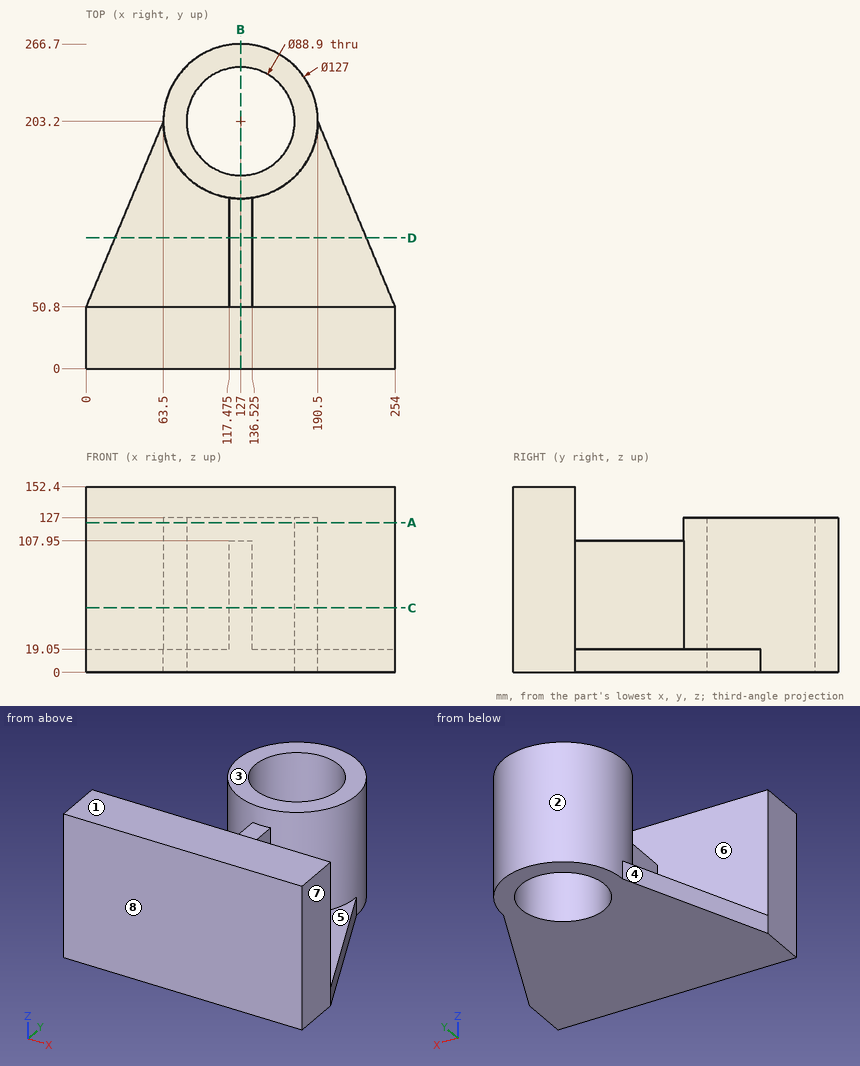
Source: three-view drawing plus pictorial views. Frame: mm from the lowest corner of the part. A direction names the side the tool comes from. Round coordinates to 2 decimals unless told otherwise and drop trailing zeros. Loops run counter-clockwise (first coordinate to the right, second up) from the corner with the lowest first, then second, coordinate; pieces in that order, holes last.
Q1. Section D-D, the plane y = 107.5. Return loops of the section in (x, z) (3 decimals), plus the area to 3 significant figures.
Q2. Section C-C, the plane z = 53. Return loops of the section in (x, y) (3 decimals), plus the area to 3 significant figures.
Q3. Ray query, line 1 (Y direction, x = 127, z = 57); line 2 (Y direction, x = 148, z = 51.5); line 3 (X direction, y = 203, z = 83). Return the intervals inside material, ascending.
Q4. Access query for the marked faces 1, 2, 3, 4 and 5. Directions: +Z, -Z, +X, -X, +Y, -Y. A direction counts if a zero-diameter tool reaches every point of the face in a straight line with its end or side. Return the directions, or none.
Q5. First-contact query: P1, Ø4, axis at y = 174, z = 99.5, coming from the -X side; P2, Ø2, axis at x = 82.5, y = 159, coming from the +Z side; P3, Ø12, axis at x = 208.5, z = 47, coming from the +Y side. Flat tips, straight axial feed; report the tip coordinate or a pass-through.
Q6. Section B-B, the plane x = 127. Return loops of the section in (y, z).
Q7. Section A-A, the plane z = 123. Return loops of the section in (x, y), plus the area to 3 significant figures.
Q8. Mould query, pull axis Y, two halves, no side actions, for the marked faces 6, 7 and 8. Classes: pulls with the +Y half, pulls with the -Y half, needs draft (parallel to the pull), parting line crosses it, or undercut.
Solutions:
1. outline: (23.625, 0) - (230.375, 0) - (230.375, 19.05) - (136.525, 19.05) - (136.525, 107.95) - (117.475, 107.95) - (117.475, 19.05) - (23.625, 19.05) - close
1. area: 5,630 mm2
2. outline: (0, 0) - (254, 0) - (254, 50.8) - (136.525, 50.8) - (136.525, 140.418) arc R63.5 ccw (long way) to (117.475, 140.418) - (117.475, 50.8) - (0, 50.8) - close; hole circle Ø88.9 at (127, 203.2)
2. area: 21,100 mm2
3. line 1: y = 0 to 158.75, 247.65 to 266.7
3. line 2: y = 0 to 50.8, 143.27 to 164.02, 242.38 to 263.13
3. line 3: x = 63.5 to 82.55, 171.45 to 190.5
4. face 1: +Z, +X, -X, +Y, -Y
4. face 2: +Z
4. face 3: +Z, +X, -X, +Y
4. face 4: +Z, -Z, -X, +Y
4. face 5: +Z, +X
5. P1: stops at x = 69.62
5. P2: stops at z = 127
5. P3: stops at y = 50.8
6. outline: (0, 0) - (158.75, 0) - (158.75, 127) - (139.7, 127) - (139.7, 107.95) - (50.8, 107.95) - (50.8, 152.4) - (0, 152.4) - close; (247.65, 0) - (266.7, 0) - (266.7, 127) - (247.65, 127) - close
7. outline: (0, 0) - (254, 0) - (254, 50.8) - (0, 50.8) - close; circle Ø127 at (127, 203.2); hole circle Ø88.9 at (127, 203.2)
7. area: 19,400 mm2
8. face 6: undercut
8. face 7: needs draft
8. face 8: pulls with the -Y half
